```python
from build123d import *

# Parameters (mm, degrees)
BOSS_EXTRUDE1_DEPTH = 3.175
FILLET1_R           = 1.27


with BuildPart() as part:
    # Sketch1 → Boss-Extrude1 (new body)
    with BuildSketch(Plane.XY):
        Polygon((35.620689733, 40.579771036), (38.795689733, 40.579771036), (38.795689733, 69.2403508), (95.945689733, 69.2403508), (95.945689733, 40.579771036), (99.120689733, 40.579771036), (99.120689733, 12.004771036), (95.945689733, 12.004771036), (95.945689733, -16.570228964), (99.120689733, -16.570228964), (99.120689733, -45.145228964), (95.945689733, -45.145228964), (38.795689733, -45.145228964), (35.620689733, -45.145228964), (35.620689733, -16.570228964), (38.795689733, -16.570228964), (38.795689733, 12.004771036), (35.620689733, 12.004771036), align=None)
        with BuildLine():
            Line((48.079687467, 64.1603508), (62.290689733, 64.1603508))
            ThreePointArc((62.290689733, 64.1603508), (64.086740957, 63.416402024), (64.830689733, 61.6203508))
            Line((64.830689733, 61.6203508), (64.830689733, 34.490159477))
            ThreePointArc((64.830689733, 34.490159477), (62.89755253, 32.023721246), (60.040675918, 33.311584986))
            Line((60.040675918, 33.311584986), (45.829673652, 60.441776309))
            ThreePointArc((45.829673652, 60.441776309), (45.90653547, 62.935269199), (48.079687467, 64.1603508))
        make_face(mode=Mode.SUBTRACT)
        with BuildLine():
            Line((69.910689733, 61.6203508), (69.910689733, 34.490159477))
            ThreePointArc((69.910689733, 34.490159477), (71.843826936, 32.023721246), (74.700703548, 33.311584986))
            Line((74.700703548, 33.311584986), (88.911705815, 60.441776309))
            ThreePointArc((88.911705815, 60.441776309), (88.834843997, 62.935269199), (86.661691999, 64.1603508))
            Line((86.661691999, 64.1603508), (72.450689733, 64.1603508))
            ThreePointArc((72.450689733, 64.1603508), (70.654638509, 63.416402024), (69.910689733, 61.6203508))
        make_face(mode=Mode.SUBTRACT)
        with BuildLine():
            Line((43.875689733, 42.900802499), (43.875689733, 15.9003508))
            ThreePointArc((43.875689733, 15.9003508), (44.619638509, 14.104299576), (46.415689733, 13.3603508))
            Line((46.415689733, 13.3603508), (60.558733389, 13.3603508))
            ThreePointArc((60.558733389, 13.3603508), (62.731885387, 14.585432401), (62.808747205, 17.078925291))
            Line((62.808747205, 17.078925291), (48.665703548, 44.07937699))
            ThreePointArc((48.665703548, 44.07937699), (45.808826936, 45.36724073), (43.875689733, 42.900802499))
        make_face(mode=Mode.SUBTRACT)
        with BuildLine():
            Line((71.932632262, 17.078925291), (86.075675918, 44.07937699))
            ThreePointArc((86.075675918, 44.07937699), (88.93255253, 45.36724073), (90.865689733, 42.900802499))
            Line((90.865689733, 42.900802499), (90.865689733, 15.9003508))
            ThreePointArc((90.865689733, 15.9003508), (90.121740957, 14.104299576), (88.325689733, 13.3603508))
            Line((88.325689733, 13.3603508), (74.182646077, 13.3603508))
            ThreePointArc((74.182646077, 13.3603508), (72.00949408, 14.585432401), (71.932632262, 17.078925291))
        make_face(mode=Mode.SUBTRACT)
        with BuildLine():
            Line((57.210689733, 10.8203508), (77.530689733, 10.8203508))
            ThreePointArc((77.530689733, 10.8203508), (79.326740957, 10.076402024), (80.070689733, 8.2803508))
            Line((80.070689733, 8.2803508), (80.070689733, -18.725228972))
            ThreePointArc((80.070689733, -18.725228972), (79.326740957, -20.521280196), (77.530689733, -21.265228972))
            Line((77.530689733, -21.265228972), (57.210689733, -21.265228972))
            ThreePointArc((57.210689733, -21.265228972), (55.414638509, -20.521280196), (54.670689733, -18.725228972))
            Line((54.670689733, -18.725228972), (54.670689733, 8.2803508))
            ThreePointArc((54.670689733, 8.2803508), (55.414638509, 10.076402024), (57.210689733, 10.8203508))
        make_face(mode=Mode.SUBTRACT)
        Polygon((42.432285336, -11.806981605), (42.432285336, -40.525537031), (54.020897102, -40.525537031), align=None, mode=Mode.SUBTRACT)
        Polygon((92.30909413, -40.525537031), (80.720482364, -40.525537031), (92.30909413, -11.806981605), align=None, mode=Mode.SUBTRACT)
    extrude(amount=BOSS_EXTRUDE1_DEPTH)

    # Fillet1
    fillet1_edges = [part.edges().sort_by_distance(p)[0] for p in [
        (54.020897102, -40.525537031, 1.5875),
        (42.432285336, -11.806981605, 1.5875),
        (42.432285336, -40.525537031, 1.5875),
        (92.30909413, -40.525537031, 1.5875),
        (92.30909413, -11.806981605, 1.5875),
        (80.720482364, -40.525537031, 1.5875),
    ]]
    fillet(fillet1_edges, radius=FILLET1_R)


solid = part.part
```
Input: part model. Units: mm. Frame: model coordinates. A direction names the side the tool comes from. Round coordinates to 2 decimals unless told otherwise and drop trailing zeros. Loops run counter-clockwise (first coordinate to the right, second up) from the corner with the lowest first, then second, coordinate; pieces in that order, holes last. Notation, with made-up numbers: (-23.75, -5.5) - (17.25, -5.5) arc R17 ccw to (17.25, 24.5) - close; hole circle Ø4 at (56, 3). An arc over 180 degrees is marked (long way). One line per item, written item: value. Start each with the question number.
(1) Draft query along Y for faces 5 (the cylindrical face through (64.067, 63.436, 1.565)), 6 (the flat face through (67, 69.24, 2)), 7 (the flat face through (99.121, -31, 2)). Return one class per face: +Y half, -Y half, draft (parallel to the pull), parting line (faces both ways), or undercut.
(2) Ray query, line 1 (Y direction, x = 69, z = 0.55); line 2 (X direction, y = -1, z = 1.25); line 3 (X direction, y = -35.5, z = 2.5). Return the intervals inside material, ascending. Write a range as [from, to].
(3) Access query for faces 1 (the flat face through (55.836, 30.39, 1.565)), 2 (the flat face through (38.796, 55, 2)), 3 (the flat face through (35.621, 26, 2)), 4 (the flat face through (37, -16.57, 2)). Directions: +Z, -Z, +X, -X, +Y, -Y. A direction counts if a zero-diameter tool reaches every point of the face in a straight line with its end or side. Return the directions, or none.
(4) Section A-A, the plane y = 1.5. Return loops of the section in (x, z) (3 decimals), plus the area to 3 significant figures.
(5) Section B-B, the plane y = 53.5. Return loops of the section in (x, z) (3 decimals).
(6) Section D-D, the plane y = 24.5. Return loops of the section in (x, z) (3 decimals), plus the area to 3 significant figures.
(7) Section C-C, the plane z = 1.2. Count the separate pieces of the cut face and the enclosed holes in it, plus the area to 3 significant figures.
(8) Contact query for flat-ended pins moving along their axis: P1, Ø1.6, axis at y = 45, z = 2, coming from the -X side; P2, Ø1.6, axis at x = 97, z = 1, coming from the +Y side; P3, Ø1, axis at y = 3.5, z = 2, coming from the +X side; P4, Ø10, axis at x = 74.5, y = -16.5, coming from the +Z side (3 decimals). Output: stop coordinate, or through.
Results below:
1. face 5: undercut
1. face 6: +Y half
1. face 7: draft
2. line 1: [-45.15, -21.27], [10.82, 69.24]
2. line 2: [38.8, 54.67], [80.07, 95.95]
2. line 3: [35.62, 42.43], [51.99, 82.75], [92.31, 99.12]
3. face 1: +Z, -Z
3. face 2: +Z, -Z, -X, +Y
3. face 3: +Z, -Z, -X, +Y, -Y
3. face 4: +Z, -Z, -X
4. outline: (38.796, 0) - (54.671, 0) - (54.671, 3.175) - (38.796, 3.175) - close; (80.071, 0) - (95.946, 0) - (95.946, 3.175) - (80.071, 3.175) - close
4. area: 101 mm^2
5. outline: (38.796, 0) - (49.466, 0) - (49.466, 3.175) - (38.796, 3.175) - close; (64.831, 0) - (69.911, 0) - (69.911, 3.175) - (64.831, 3.175) - close; (85.276, 0) - (95.946, 0) - (95.946, 3.175) - (85.276, 3.175) - close
6. outline: (35.621, 0) - (43.876, 0) - (43.876, 3.175) - (35.621, 3.175) - close; (58.922, 0) - (75.82, 0) - (75.82, 3.175) - (58.922, 3.175) - close; (90.866, 0) - (99.121, 0) - (99.121, 3.175) - (90.866, 3.175) - close
6. area: 106 mm^2
7. separate pieces: 1
7. enclosed holes: 7
7. area: 4,190 mm^2
8. P1: x = 38.8
8. P2: y = 40.58
8. P3: x = 95.95
8. P4: z = 3.175
